Autodesk Inventor part; units mm, degrees
ref_plane "YZ Plane" through (0, 0, 0) normal (1, 0, 0) x (0, 1, 0)
ref_plane "XZ Plane" through (0, 0, 0) normal (0, 1, 0) x (-1, 0, 0)
ref_plane "XY Plane" through (0, 0, 0) normal (0, 0, 1) x (1, 0, 0)
sketch "Sketch1" plane through (0, 0, 0) normal (0, 1, 0) x (-1, 0, 0)
  circle A0 centre (0, 0) radius 4.5
  dimension "d0" = 9
extrude "Extrusion1" add sketch "Sketch1" along normal blind 2
chamfer "Chamfer1" distance 2.5 distance2 2 1 edges at (4.5, 2, 0) measured on face at (-0.1808, 2, 1.316)
sketch "Sketch2" plane through (0, 2, 0) normal (0, 1, 0) x (1, 0, 0)
  circle A0 centre (0, 0) radius 2
extrude "Extrusion2" add sketch "Sketch2" along normal blind 18
properties part number "pulley screw"
Check sheet for the modelled part. Datum: model origin and axes. Units: mm. A direction names the side the tool comes from. Round coordinates to 2 decimals unless told otherwise and drop trailing zeros. Order: outer loops, then holes, each group sorted by start corner. A loop starts at its lowest first (then second) coordinate and runs counter-clockwise, first axis right, second up. Notation, with made-up numbers: (47.5, 7.5) -> (66.5, 7.5) arc R33 ccw to (66.5, 42.5) -> close; hole circle Ø2 at (-2, -36.75). An arc over 180 degrees is marked (long way). Use CSV: the item, a comma, the result in double quotes.
(1) Tool access check on faces 1 (the face through (0, 20, 0)), 2 (the face through (0, 11, -2)). Record the directions out of +Z, -Z, +X, -X, +Y, -Y that give a thin tool (end or side, any length) a straight path to the whole face; none if there is none.
Worked out:
face 1,"+Z, -Z, +X, -X, +Y"
face 2,"+Y"
(2) Material ranges on line 1 along Z through (x, y) = (0, 3.75); line 2 along Y through (x, z) = (-3.25, 0.75); line 3 along Y through (x, z) = (3.75, -0.75), recorded low to high. Write a range as from..to.
Worked out:
line 1,"-2..2"
line 2,"0..0.93"
line 3,"0..0.54"
(3) Cross-section at C-C (y = 17). Record the boundary of the cut face in (x, z), and give its area (3 significant figures).
Worked out:
outline,"circle Ø4 at (0, 0)"
area,"12.6 mm²"
(4) Depth check by flat-ended pin: pin 1 (4 mm diameter, centred on y = 13, z = 3, fed in from -X); pin 2 (2 mm diameter, centred on x = -0.5, y = 4.5, fed in from -Z). Enter the tip coordinate at first touch or a pass-through.
Worked out:
pin 1,"x = -1.73"
pin 2,"z = -2"
